```python
from build123d import *

# Parameters (mm, degrees)
F0_W     = 30
F0_H     = 40
F0_W_2   = 14
F0_H_2   = 36
F1_DEPTH = 70
F2_DEPTH = 7
F3_R     = 3
F4_DEPTH = 15
F6_DEPTH = 5


with BuildPart() as f1:
    # F0 (on Top) → F1 (new body)
    with BuildSketch(Plane.XY):
        Rectangle(F0_W, F0_H)
        with Locations((2, 0)):
            Rectangle(F0_W_2, F0_H_2, mode=Mode.SUBTRACT)
        with Locations((2, 0)):
            Rectangle(F0_W_2, F0_H_2)
    extrude(amount=F1_DEPTH)

    # F0 (on Top) → F2 (join)
    with BuildSketch(Plane.XY):
        with Locations((2, 0)):
            Rectangle(F0_W_2, F0_H_2)
    extrude(amount=-F2_DEPTH)

    # F3 (on face) → F4 (join)
    with BuildSketch(Plane.XY.offset(70)):
        with Locations((2, -14)):
            Circle(F3_R)
    extrude(amount=F4_DEPTH)

    # F5 (on face) → F6 (cut)
    with BuildSketch(Plane(origin=(-15, 0, 0), x_dir=(0, -1, 0), z_dir=(-1, 0, 0))):
        with BuildLine():
            ThreePointArc((9, 15), (10, 14), (11, 15))
            ThreePointArc((11, 15), (10, 16), (9, 15))
        make_face()
        with BuildLine():
            ThreePointArc((9, 15), (10, 16), (11, 15))
            Line((11, 15), (11, 31))
            ThreePointArc((11, 31), (10, 30), (9, 31))
            Line((9, 31), (9, 15))
        make_face()
        with BuildLine():
            ThreePointArc((9, 31), (10, 30), (11, 31))
            ThreePointArc((11, 31), (10, 32), (9, 31))
        make_face()
        with BuildLine():
            ThreePointArc((9, 55), (10, 54), (11, 55))
            ThreePointArc((11, 55), (10, 56), (9, 55))
        make_face()
        with BuildLine():
            ThreePointArc((4, 55), (5, 54), (6, 55))
            ThreePointArc((6, 55), (5, 56), (4, 55))
        make_face()
        with BuildLine():
            ThreePointArc((-1, 55), (0, 54), (1, 55))
            ThreePointArc((1, 55), (0, 56), (-1, 55))
        make_face()
        with BuildLine():
            ThreePointArc((-6, 55), (-5, 54), (-4, 55))
            ThreePointArc((-4, 55), (-5, 56), (-6, 55))
        make_face()
        with BuildLine():
            ThreePointArc((-11, 55), (-10, 54), (-9, 55))
            ThreePointArc((-9, 55), (-10, 56), (-11, 55))
        make_face()
        with BuildLine():
            ThreePointArc((9, 39), (10, 40), (11, 39))
            Line((11, 39), (11, 55))
            ThreePointArc((11, 55), (10, 54), (9, 55))
            Line((9, 55), (9, 39))
        make_face()
        with BuildLine():
            ThreePointArc((4, 39), (5, 40), (6, 39))
            Line((6, 39), (6, 55))
            ThreePointArc((6, 55), (5, 54), (4, 55))
            Line((4, 55), (4, 39))
        make_face()
        with BuildLine():
            ThreePointArc((-1, 39), (0, 40), (1, 39))
            Line((1, 39), (1, 55))
            ThreePointArc((1, 55), (0, 54), (-1, 55))
            Line((-1, 55), (-1, 39))
        make_face()
        with BuildLine():
            ThreePointArc((-6, 39), (-5, 40), (-4, 39))
            Line((-4, 39), (-4, 55))
            ThreePointArc((-4, 55), (-5, 54), (-6, 55))
            Line((-6, 55), (-6, 39))
        make_face()
        with BuildLine():
            ThreePointArc((-11, 39), (-10, 40), (-9, 39))
            Line((-9, 39), (-9, 55))
            ThreePointArc((-9, 55), (-10, 54), (-11, 55))
            Line((-11, 55), (-11, 39))
        make_face()
        with BuildLine():
            ThreePointArc((9, 39), (10, 38), (11, 39))
            ThreePointArc((11, 39), (10, 40), (9, 39))
        make_face()
        with BuildLine():
            ThreePointArc((4, 39), (5, 38), (6, 39))
            ThreePointArc((6, 39), (5, 40), (4, 39))
        make_face()
        with BuildLine():
            ThreePointArc((-1, 39), (0, 38), (1, 39))
            ThreePointArc((1, 39), (0, 40), (-1, 39))
        make_face()
        with BuildLine():
            ThreePointArc((-6, 39), (-5, 38), (-4, 39))
            ThreePointArc((-4, 39), (-5, 40), (-6, 39))
        make_face()
        with BuildLine():
            ThreePointArc((-11, 39), (-10, 38), (-9, 39))
            ThreePointArc((-9, 39), (-10, 40), (-11, 39))
        make_face()
        with BuildLine():
            ThreePointArc((4, 31), (5, 30), (6, 31))
            ThreePointArc((6, 31), (5, 32), (4, 31))
        make_face()
        with BuildLine():
            ThreePointArc((-1, 31), (0, 30), (1, 31))
            ThreePointArc((1, 31), (0, 32), (-1, 31))
        make_face()
        with BuildLine():
            ThreePointArc((-6, 31), (-5, 30), (-4, 31))
            ThreePointArc((-4, 31), (-5, 32), (-6, 31))
        make_face()
        with BuildLine():
            ThreePointArc((-11, 31), (-10, 30), (-9, 31))
            ThreePointArc((-9, 31), (-10, 32), (-11, 31))
        make_face()
        with BuildLine():
            ThreePointArc((4, 15), (5, 16), (6, 15))
            Line((6, 15), (6, 31))
            ThreePointArc((6, 31), (5, 30), (4, 31))
            Line((4, 31), (4, 15))
        make_face()
        with BuildLine():
            ThreePointArc((-1, 15), (0, 16), (1, 15))
            Line((1, 15), (1, 31))
            ThreePointArc((1, 31), (0, 30), (-1, 31))
            Line((-1, 31), (-1, 15))
        make_face()
        with BuildLine():
            ThreePointArc((-6, 15), (-5, 16), (-4, 15))
            Line((-4, 15), (-4, 31))
            ThreePointArc((-4, 31), (-5, 30), (-6, 31))
            Line((-6, 31), (-6, 15))
        make_face()
        with BuildLine():
            ThreePointArc((-11, 15), (-10, 16), (-9, 15))
            Line((-9, 15), (-9, 31))
            ThreePointArc((-9, 31), (-10, 30), (-11, 31))
            Line((-11, 31), (-11, 15))
        make_face()
        with BuildLine():
            ThreePointArc((4, 15), (5, 14), (6, 15))
            ThreePointArc((6, 15), (5, 16), (4, 15))
        make_face()
        with BuildLine():
            ThreePointArc((-1, 15), (0, 14), (1, 15))
            ThreePointArc((1, 15), (0, 16), (-1, 15))
        make_face()
        with BuildLine():
            ThreePointArc((-6, 15), (-5, 14), (-4, 15))
            ThreePointArc((-4, 15), (-5, 16), (-6, 15))
        make_face()
        with BuildLine():
            ThreePointArc((-11, 15), (-10, 14), (-9, 15))
            ThreePointArc((-9, 15), (-10, 16), (-11, 15))
        make_face()
    extrude(amount=-F6_DEPTH, mode=Mode.SUBTRACT)


solid = f1.part
```
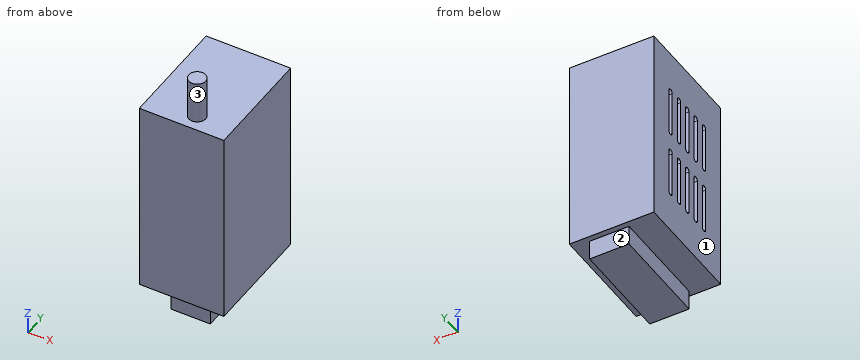
Geometry check sheet. Reference: the model listing, model coordinates, mm. Face numbers are marked on the shaded views. A direction names the side the tool comes from. Round coordinates to 2 decimals unless told otherwise and drop trailing zeros. Loops run counter-clockwise (first coordinate to the right, second up) from the corner with the lowest first, then second, coordinate; pieces in that order, holes last. Notation, with made-up numbers: (-20, -15.75) - (38, -15.75) arc R27 cw to (38, 2.25) - close; hole circle Ø8 at (74.25, 17). An arc over 180 degrees is marked (long way). Write item = value, one per line. Start each with the question number.
1. Thickness scan on line 1 (Z direction, x = -11.25, y = 5); line 2 (Y direction, x = -12, z = 15); line 3 (Z direction, x = -13, y = -1.5). Record the ranges inside material, lowest first.
2. Section check C-C on z = 47.5. Enter the section's corners in (x, y).
3. Depth check by flat-ended pin: pin 1 (1.6 mm diameter, centred on y = -5, z = 26.5, fed in from -X); pin 2 (3.5 mm diameter, centred on x = 5, z = -3.5, fed in from +Y); pin 3 (5.5 mm diameter, centred on y = 3, z = -4.5, fed in from +X). Enter the tip coordinate at first touch or a pass-through.
4. Section check A-A on y = 0. Enter the section's corners in (x, z), then the cut area to 3 significant figures.
5. Set-up check for the marked faces 1, 2 and 3: record each of +Z, -Z, +X, -X, +Y, -Y from which the full face is reachable in a straight line by a thin tool's end or side.
6. Section check B-B on x = 2. Enter the section's corners in (y, z).
7. Section check D-D on y = -14. Enter the section's corners in (x, z).
Working result:
q1.line_1 = 0 to 14, 32 to 38, 56 to 70
q1.line_2 = -20 to -11, -9 to -6, -4 to -1, 1 to 4, 6 to 9, 11 to 20
q1.line_3 = 0 to 70
q2.outline = (-15, -20) - (15, -20) - (15, 20) - (-15, 20) - (-15, 11) - (-10, 11) - (-10, 9) - (-15, 9) - (-15, 6) - (-10, 6) - (-10, 4) - (-15, 4) - (-15, 1) - (-10, 1) - (-10, -1) - (-15, -1) - (-15, -4) - (-10, -4) - (-10, -6) - (-15, -6) - (-15, -9) - (-10, -9) - (-10, -11) - (-15, -11) - close
q3.pin_1 = -10
q3.pin_2 = 18
q3.pin_3 = 9
q4.outline = (-15, 0) - (-5, 0) - (-5, -7) - (9, -7) - (9, 0) - (15, 0) - (15, 70) - (-15, 70) - (-15, 56) - (-10, 56) - (-10, 38) - (-15, 38) - (-15, 32) - (-10, 32) - (-10, 14) - (-15, 14) - close
q4.area = 2,020 mm^2
q5.face_1 = +Z, -Z, -X, +Y, -Y
q5.face_2 = -Z, +X, -X, +Y
q5.face_3 = +Z
q6.outline = (-20, 0) - (-18, 0) - (-18, -7) - (18, -7) - (18, 0) - (20, 0) - (20, 70) - (-11, 70) - (-11, 85) - (-17, 85) - (-17, 70) - (-20, 70) - close
q7.outline = (-15, 0) - (-5, 0) - (-5, -7) - (9, -7) - (9, 0) - (15, 0) - (15, 70) - (5, 70) - (5, 85) - (-1, 85) - (-1, 70) - (-15, 70) - close
